Design review of the part built by this model. Coordinates are the model's own, in mm. A direction names the side the tool comes from. Round coordinates to 2 decimals unless told otherwise and drop trailing zeros. Write each loop counter-clockwise with the first axis right and the second up, starting at its lowest first coordinate (ties: lowest second). Pieces come first, ordered by that corner, then holes.
from build123d import *

# Parameters (mm, degrees)
SKETCH029_W  = 6
SKETCH029_H  = 3.8
PAD012_DEPTH = 2
SKETCH033_R  = 1.9
PAD016_DEPTH = 15.4
FILLET012_R  = 1


with BuildPart() as part:
    # Sketch029 → Pad012 (new body)
    with BuildSketch(Plane.XY.offset(13.4)):
        with Locations((1.7, -30.5)):
            Rectangle(SKETCH029_W, SKETCH029_H)
    extrude(amount=PAD012_DEPTH)

    # Sketch033 (on Face5 of Pad012) → Pad016 (join)
    with BuildSketch(Plane(origin=(0, 0, 13.4), x_dir=(1, 0, 0), z_dir=(0, 0, -1))):
        with Locations((1.7, 30.5)):
            Circle(SKETCH033_R)
    extrude(amount=PAD016_DEPTH)

    # Fillet012
    fillet012_edges = [part.edges().sort_by_distance(p)[0] for p in [
        (-0.2, -30.5, -2),
    ]]
    fillet(fillet012_edges, radius=FILLET012_R)


solid = part.part
1) Add section B-B on z = -0.5. State the section outline as (x, y) points, and give its area (3 significant figures).
2) Add section A-A on x = 4.1. State the section outline as (y, z) points.
3) For faces 1 (the face through (4, -30, 13.4)), 2 (the face through (1.453, -32.384, 6.301)), 3 (the face through (-0.5, -30.5, 13.4)), list the 3-axis set-ups (+Z, -Z, +X, -X, +Y, -Y) from which the entire face can be reached by the end or side of a thin tool; tool diameter is ignored.
4) For P1, Ø2, axis at y = -29.5, z = 3, coming from the -X side, flat-tipped, find the tip position at first contact; note if it passes through.
5) For line 1 along Z through (x, y) = (3.9, -30); line 2 along Y through (x, z) = (1.6, 7.75); line 3 along X through (y, z) = (-30.5, 4.25), list the stretches that pass through material, from the lowest coordinate up.
Computed:
1. outline: circle Ø3.8 at (1.7, -30.5)
1. area: 11.3 mm2
2. outline: (-32.4, 13.4) - (-28.6, 13.4) - (-28.6, 15.4) - (-32.4, 15.4) - close
3. face 1: -Z, +X
3. face 2: -Z
3. face 3: -Z, -X
4. P1: stops at x = -0.2
5. line 1: z = 13.4 to 15.4
5. line 2: y = -32.4 to -28.6
5. line 3: x = -0.2 to 3.6
